For this review, take the finished solid that the model builds, in its own axes (mm). A direction names the side the tool comes from. Coordinates: 2 decimals unless noted, no trailing zeros. Loops run counter-clockwise (first coordinate to the right, second up) from the corner with the lowest first, then second, coordinate; pieces in that order, holes last. Notation, with made-up numbers: M 15.5,63.25 L 32.5,63.25 A33 ccw 32.5,92.25 Z; hole C 80,-6.5 d11. An arc over 180 degrees is marked long. Use one line per item in the form item = value.
Autodesk Inventor part; units mm, degrees
ref_plane "YZ Plane" through (0, 0, 0) normal (1, 0, 0) x (0, 1, 0)
ref_plane "XZ Plane" through (0, 0, 0) normal (0, 1, 0) x (-1, 0, 0)
ref_plane "XY Plane" through (0, 0, 0) normal (0, 0, 1) x (1, 0, 0)
sketch "Sketch1" plane through (0, 0, 0) normal (0, 1, 0) x (-1, 0, 0)
  line L0 (0, 0) -> (305, 0)
  line L1 (305, 0) -> (305, -10)
  line L2 (305, -10) -> (0, -10)
  line L3 (0, -10) -> (0, 0)
  dimension "d0" = 305
  dimension "d1" = 10
extrude "Extrusion1" add sketch "Sketch1" along normal blind 40
sketch "Sketch2" plane through (-305, 0, 0) normal (0, 0, 1) x (1, 0, 0)
  line L0 (305, 0) -> (0, 0)
  line L1 (305, 0) -> (305, 40)
  line L2 (0, 0) -> (305, 0)
  line L3 (305, 0) -> (305, 8)
  line L4 (305, 8) -> (0, 8)
  line L5 (0, 8) -> (0, 0)
  dimension "d4" = 8
extrude "Extrusion2" add sketch "Sketch2" along normal blind 20
sketch "Sketch3" plane through (-305, 40, 0) normal (0, 0, 1) x (1, 0, 0)
  line L0 (305, -27) -> (0, -27)
  line L1 (5, -5) -> (300, -5)
  line L2 (300, -5) -> (300, -27)
  line L3 (300, -27) -> (5, -27)
  line L4 (5, -27) -> (5, -5)
  line L5 (0, -32) -> (0, 0)
  line L6 (0, 0) -> (305, 0)
  line L7 (305, -32) -> (305, 0)
  point P0 (305, -40)
  point P1 (305, -16)
  dimension "d8" = 5
  dimension "d9" = 5
  dimension "d10" = 5
extrude "Extrusion3" cut sketch "Sketch3" against normal blind 20 contours L0 L4 L1 L2
fillet "Fillet2" radius 5 4 edges at (-300, 13, -5) (-300, 35, -5) (-5, 13, -5) (-5, 35, -5)
sketch "Sketch4" plane through (-305, 0, -10) normal (-1, 0, 0) x (0, 0, 1)
  circle A0 centre (5, 25) radius 1.5
  circle A1 centre (5, 12) radius 1.5
  line L0 (0, 40) -> (10, 40)
  line L1 (0, 0) -> (0, 40)
  point P0 (10, 0)
  dimension "d14" = 3
  dimension "d15" = 3
  dimension "d16" = 15
  dimension "d17" = 10
  dimension "d18" = 5
  dimension "d19" = 5
extrude "Extrusion4" cut sketch "Sketch4" against normal blind 20
sketch "Sketch5" plane through (0, 0, -10) normal (1, 0, 0) x (0, 0, -1)
  circle A0 centre (-5, 25) radius 1.5
  circle A1 centre (-5, 12) radius 1.5
  line L0 (0, 0) -> (0, 40)
  line L1 (-10, 40) -> (0, 40)
  point P0 (-10, 0)
  dimension "d22" = 3
  dimension "d23" = 3
  dimension "d24" = 5
  dimension "d25" = 5
  dimension "d26" = 10
  dimension "d27" = 15
extrude "Extrusion5" cut sketch "Sketch5" against normal blind 20
thread "Thread1"
thread "Thread2"
thread "Thread3"
thread "Thread4"
properties part number "chessboard-base-2"
1. Consider section A-A on x = -122. Write out the cut boundary in (y, z), plus the area to 3 significant figures.
Computed values:
outline = M 0,-10 L 13,-10 L 13,0 L 8,0 L 8,20 L 0,20 Z; M 35,-10 L 40,-10 L 40,0 L 35,0 Z
area = 340 mm2
2. Tool access review of faces 5 (the face through (-150, 40, -5)), 6 (the face through (-154, 35, -5)), 7 (the face through (-140, 12, 0)): name each direction out of +Z, -Z, +X, -X, +Y, -Y from which nothing blocks a thin tool from reaching the whole face with its end or side.
Computed values:
face_5 = +Z, -Z, +X, -X, +Y
face_6 = +Z, -Z
face_7 = +Z, +X, -X, +Y
3. Consider section B-B on z = 12. Write out the cut boundary in (x, y).
Computed values:
outline = M -305,0 L 0,0 L 0,8 L -305,8 Z
4. For pin 1 Ø10 at (x, z) = (-164.5, 6) entering from +Y; pin 2 Ø8 at (y, z) = (17.5, 6) entering from -X; pin 3 Ø0.8 at (y, z) = (12, -4.5) entering from +X, all flat-tipped, find the tip position at first contact; note any pin that passes through.
Computed values:
pin_1 = 8
pin_2 = through
pin_3 = -20
5. Draft analysis for pull direction Y (two halves, no side actions). For faces 1 (the face through (-150, 8, 10)), 2 (the face through (-150, 0, 5)), 3 (the face through (-5, 23, -5)), 4 (the face through (-305, 15, -1)), state which applies: +Y half, -Y half, draft (parallel to the pull), parting line (faces both ways), or undercut.
Computed values:
face_1 = +Y half
face_2 = -Y half
face_3 = undercut
face_4 = draft
6. Wall thickness on line 1 along Y through (x, z) = (-302.6, -5); line 2 along Y through (x, z) = (-169.5, -7); line 3 along Y through (x, z) = (-7, -5): over which ranges is each line inside the solid? List them lowest first. Write a range as from..to.
Computed values:
line_1 = 0..10.5, 13.5..23.5, 26.5..40
line_2 = 0..13, 35..40
line_3 = 0..10.5, 13.5..14, 34..40
